The listing builds one solid part. Answer for the finished solid, in the listing's coordinates (mm). Face numbers are marked on the shaded views. A direction names the side the tool comes from. Give positions to 0.01 mm unless a question says otherwise; leave off trailing zeros. Loops run counter-clockwise (first coordinate to the right, second up) from the corner with the lowest first, then second, coordinate; pieces in that order, holes last. Notation, with made-up numbers: M -8,50.25 L 34,50.25 A14 ccw 34,55.25 Z; hole C -7,54.5 d7. An arc over 180 degrees is marked long. Return JSON: item names as keys, results as strings.
from build123d import *

# Parameters (mm, degrees)
SKETCH_1_R      = 1.5
EXTRUDE_1_DEPTH = 4


with BuildPart() as part:
    # Эскиз1 → Бобышка-Вытянуть1 (new body)
    with BuildSketch(Plane.XY):
        Polygon((0, 0), (5, 0), (5, -4), (15, -4), (15, 0), (20, 0), (20, 13.5), (16, 13.5), (16, 23.5), (20, 23.5), (20, 37), (15, 37), (15, 41), (5, 41), (5, 37), (0, 37), (0, 23.5), (4, 23.5), (4, 13.5), (0, 13.5), align=None)
        with Locations((10, 23.5)):
            Circle(SKETCH_1_R, mode=Mode.SUBTRACT)
        with Locations(Location((10, 13.5, 0), (0, 0, 180))):
            Circle(SKETCH_1_R, mode=Mode.SUBTRACT)
    extrude(amount=EXTRUDE_1_DEPTH)


solid = part.part
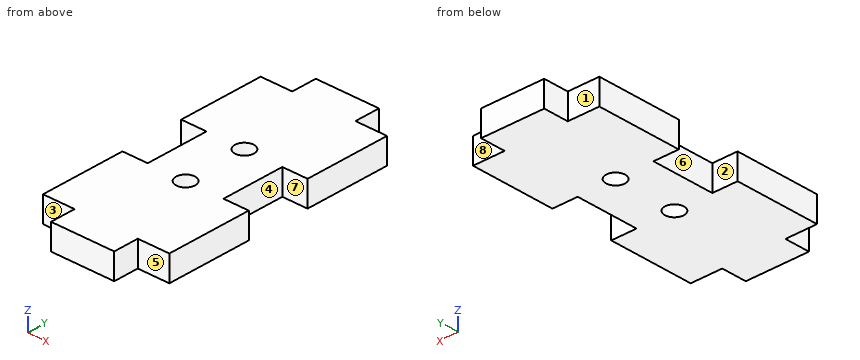
(1) Straight lines are drawn through the part: line 1 along Y through (x, z) = (10, 2.6); line 2 along Y through (x, z) = (11.25, 1.2); line 3 along Y through (x, z) = (2, 3.35). For each, find the intervals that lie inside material, in ascending order.
Values follow:
{"line 1": "-4 to 12, 15 to 22, 25 to 41", "line 2": "-4 to 12.67, 14.33 to 22.67, 24.33 to 41", "line 3": "0 to 13.5, 23.5 to 37"}
(2) Given pin 1 (2 mm diameter, centred on x = 19, z = 2.5, fed in from +Y); pin 2 (2 mm diameter, centred on y = -2.5, z = 2, fed in from -X); pin 3 (2 mm diameter, centred on x = 1, z = 1, fed in from -Y), each flat-ended and moving along its own axis, determine where each tip first touches the part or whether it passes through.
Values follow:
{"pin 1": "y = 37", "pin 2": "x = 5", "pin 3": "y = 0"}
(3) The part is cut by section D-D (x = 10). Determine the outline of the cut face in (y, z), and give its area (3 significant figures).
Values follow:
{"outline": "M -4,0 L 12,0 L 12,4 L -4,4 Z; M 15,0 L 22,0 L 22,4 L 15,4 Z; M 25,0 L 41,0 L 41,4 L 25,4 Z", "area": "156 mm²"}
(4) The part is cut by section B-B (y = 13). Determine the outline of the cut face in (x, z), and give its area (3 significant figures).
Values follow:
{"outline": "M 0,0 L 8.59,0 L 8.59,4 L 0,4 Z; M 11.41,0 L 20,0 L 20,4 L 11.41,4 Z", "area": "68.7 mm²"}
(5) A tool of negligible diameter and unlimited length cuts with its end or side. For the marked faces 5, 6, 7 and 8, from which of +Z, -Z, +X, -X, +Y, -Y can it reach the whole face along a straight path? Write none if from no direction.
Values follow:
{"face 5": "+Z, -Z, +X, -Y", "face 6": "+Z, -Z, -X", "face 7": "+Z, -Z, +X", "face 8": "+Z, -Z, +X, +Y"}
(6) The part is cut by section C-C (z = 1.5). Determine the outline of the cut face in (x, y), and give its area (3 significant figures).
Values follow:
{"outline": "M 0,0 L 5,0 L 5,-4 L 15,-4 L 15,0 L 20,0 L 20,13.5 L 16,13.5 L 16,23.5 L 20,23.5 L 20,37 L 15,37 L 15,41 L 5,41 L 5,37 L 0,37 L 0,23.5 L 4,23.5 L 4,13.5 L 0,13.5 Z; hole C 10,13.5 d3; hole C 10,23.5 d3", "area": "726 mm²"}
(7) Determine the mould class of the marked faces 1, 2, 3 and 4 for opening direction Y: released by +Y, released by -Y, zero draft, split by the parting line, or undercut.
Values follow:
{"face 1": "released by +Y", "face 2": "undercut", "face 3": "released by -Y", "face 4": "undercut"}
(8) The part is cut by section A-A (x = 2.5). Determine the outline of the cut face in (y, z), and give its area (3 significant figures).
Values follow:
{"outline": "M 0,0 L 13.5,0 L 13.5,4 L 0,4 Z; M 23.5,0 L 37,0 L 37,4 L 23.5,4 Z", "area": "108 mm²"}
